Model file for the job. Use its own axes, mm. A direction names the side the tool comes from. Give positions to 0.01 mm unless a question says otherwise; leave off trailing zeros. Loops run counter-clockwise (first coordinate to the right, second up) from the corner with the lowest first, then second, coordinate; pieces in that order, holes last. Notation, with made-up numbers: (45, 22.5) - (103, 22.5) arc R20 cw to (103, 34.5) - close; hole circle Ø8 at (68.5, -11). An arc over 180 degrees is marked (long way). Answer as CSV lines item,"result". Start each with the question number.
Item 1: Tool access for faces 1 (the flat face through (-3.81, -28, 65)), 2 (the flat face through (-22, 22, 7.62)), 3 (the flat face through (22, -22, 7.62)), 4 (the flat face through (22, 22, 7.62)): list every direction of +Z, -Z, +X, -X, +Y, -Y with a clear straight run to the whole face (end or side of a thin tool).
Item 2: Saw through at C-C on z = 88. Give the cut face in (x, y).
Item 3: Drill centre lines: L1, parallel to Y at x = 30, z = 101; L2, parallel to Z at x = -26.5, y = 29. Where is each one in solid material? Low to high. Write a range as from..to.
Item 4: Saw through at B-B on x = 40.5. Give the cut face in (y, z).
Item 5: Pull direction Z, two halves, no side cores. Call faces 5 (the flat face through (-3.81, 27, 65)), 6 (the flat face through (-1, 1, 0)), 7 (the cylindrical face through (-0.053, -36.88, 106.056)): pulls with the +Z half, pulls with the -Z half, needs draft (parallel to the pull), parting line crosses it, or undercut.
Item 6: Saw through at A-A on y = -14.5. Give the cut face in (x, z), plus the area to 3 significant figures.
Item 7: Saw through at D-D on z = 107. Give the cut face in (x, y), plus the area to 3 significant figures.
Item 8: Pin check, flat tips, straight feed: pin 1 (23.5 mm diameter, centred on x = -25, y = -20.5, fed in from +Z); pin 2 (2 mm diameter, centred on y = 6.5, z = 108, fed in from -X); pin 3 (14 mm diameter, centred on x = 27.5, z = 45, fed in from -Y). Stop position of each tip, or through.
from build123d import *

# Parameters (mm, degrees)
F0_R          = 50.8
F1_DEPTH      = 7.62
F3_DEPTH      = 3.81
F3_DEPTH_BACK = 3.81
F5_DEPTH      = 3.81
F5_DEPTH_BACK = 3.81
F6_R          = 73.848942
F6_R_2        = 50.8
F7_DEPTH      = 127


with BuildPart() as f1:
    # F0 (on Top) → F1 (new body)
    with BuildSketch(Plane.XY):
        Circle(F0_R)
    extrude(amount=F1_DEPTH)

    # F2 (on Front) → F3 (join, two sides)
    with BuildSketch(Plane.XZ) as f3_sk:
        with BuildLine():
            Line((50.8, 7.62), (50.8, 71.12))
            ThreePointArc((50.8, 71.12), (0, 121.92), (-50.8, 71.12))
            Line((-50.8, 71.12), (-50.8, 7.62))
            Line((-50.8, 7.62), (50.8, 7.62))
        make_face()
    extrude(amount=F3_DEPTH)
    extrude(f3_sk.sketch, amount=-F3_DEPTH_BACK)

    # F4 (on Right) → F5 (join, two sides)
    with BuildSketch(Plane.YZ) as f5_sk:
        with BuildLine():
            Line((50.8, 7.62), (50.8, 71.12))
            ThreePointArc((50.8, 71.12), (0, 121.92), (-50.8, 71.12))
            Line((-50.8, 71.12), (-50.8, 7.62))
            Line((-50.8, 7.62), (50.8, 7.62))
        make_face()
    extrude(amount=F5_DEPTH)
    extrude(f5_sk.sketch, amount=-F5_DEPTH_BACK)

    # F6 (on face) → F7 (cut)
    with BuildSketch(Plane(origin=(0, 0, 0), x_dir=(1, 0, 0), z_dir=(0, 0, -1))):
        Circle(F6_R)
        Circle(F6_R_2, mode=Mode.SUBTRACT)
    extrude(amount=-F7_DEPTH, mode=Mode.SUBTRACT)


solid = f1.part
Responses:
1,face 1,"+Z, -X, -Y"
1,face 2,"+Z, -X, +Y"
1,face 3,"+Z, +X, -Y"
1,face 4,"+Z, +X, +Y"
2,outline,"(-47.91, -3.81) - (-3.81, -3.81) - (-3.81, -47.91) - (3.81, -47.91) - (3.81, -3.81) - (47.91, -3.81) - (47.91, 3.81) - (3.81, 3.81) - (3.81, 47.91) - (-3.81, 47.91) - (-3.81, 3.81) - (-47.91, 3.81) - close"
3,L1,"-3.81..3.81"
3,L2,"0..7.62"
4,outline,"(-30.67, 0) - (30.67, 0) - (30.67, 7.62) - (3.81, 7.62) - (3.81, 101.79) - (-3.81, 101.79) - (-3.81, 7.62) - (-30.67, 7.62) - close"
5,face 5,"needs draft"
5,face 6,"pulls with the -Z half"
5,face 7,"pulls with the +Z half"
6,outline,"(-48.69, 0) - (48.69, 0) - (48.69, 7.62) - (3.81, 7.62) - (3.81, 119.81) - (-3.81, 119.81) - (-3.81, 7.62) - (-48.69, 7.62) - close"
6,area,"1,600 mm2"
7,outline,"(-35.96, -3.81) - (-3.81, -3.81) - (-3.81, -35.96) - (3.81, -35.96) - (3.81, -3.81) - (35.96, -3.81) - (35.96, 3.81) - (3.81, 3.81) - (3.81, 35.96) - (-3.81, 35.96) - (-3.81, 3.81) - (-35.96, 3.81) - close"
7,area,"1,040 mm2"
8,pin 1,"z = 7.62"
8,pin 2,"x = -3.81"
8,pin 3,"y = -3.81"
